```python
from build123d import *

# Parameters (mm, degrees)
F0_R     = 1.85
F0_R_2   = 0.5
F0_W     = 53
F0_H     = 53
F1_DEPTH = 1


with BuildPart() as f1:
    # F0 (on Top) → F1 (new body)
    with BuildSketch(Plane.XY):
        with BuildLine():
            Line((-44, -51), (44, -51))
            ThreePointArc((44, -51), (48.949747, -48.949747), (51, -44))
            Line((51, -44), (51, 44))
            ThreePointArc((51, 44), (48.949747, 48.949747), (44, 51))
            Line((44, 51), (-44, 51))
            ThreePointArc((-44, 51), (-48.949747, 48.949747), (-51, 44))
            Line((-51, 44), (-51, -44))
            ThreePointArc((-51, -44), (-48.949747, -48.949747), (-44, -51))
        make_face()
        with Locations((-41.5, -41.5)):
            Circle(F0_R, mode=Mode.SUBTRACT)
        with Locations((-35.074029, -20.25)):
            Circle(F0_R_2, mode=Mode.SUBTRACT)
        with Locations((41.5, -41.5)):
            Circle(F0_R, mode=Mode.SUBTRACT)
        with Locations((35.074029, -20.25)):
            Circle(F0_R_2, mode=Mode.SUBTRACT)
        with Locations((-41.5, 41.5)):
            Circle(F0_R, mode=Mode.SUBTRACT)
        Rectangle(F0_W, F0_H, mode=Mode.SUBTRACT)
        with Locations((0, 40.5)):
            Circle(F0_R_2, mode=Mode.SUBTRACT)
        with Locations((41.5, 41.5)):
            Circle(F0_R, mode=Mode.SUBTRACT)
    extrude(amount=F1_DEPTH)


solid = f1.part
```
Can you work these out from the model? Positions are in its coordinate system, mm. Coordinates: 2 decimals unless noted, no trailing zeros. Loops run counter-clockwise (first coordinate to the right, second up) from the corner with the lowest first, then second, coordinate; pieces in that order, holes last.
Item 1: If we mould it in two halves opening along Y, with no side actions, what happens to faces 1 (the face through (49, 48.9, 0.5)), 2 (the face through (40.032, 40.374, 0.493)), 3 (the face through (33, 1, 1))? For each: released by +Y, released by -Y, zero draft, split by the parting line, or undercut.
Answers below:
face 1: released by +Y
face 2: undercut
face 3: zero draft
Item 2: Suppose I cut it at C-C (z = 0.75). State how many separate pieces and enclosed holes the cut face has, then the cut area to 3 significant figures.
Answers below:
separate pieces: 1
enclosed holes: 8
area: 7,510 mm2
Item 3: Suppose I cut it at A-A (x = -10.5). Please give me the cut outline in (y, z), then the cut area to 3 significant figures.
Answers below:
outline: (-51, 0) - (-26.5, 0) - (-26.5, 1) - (-51, 1) - close; (26.5, 0) - (51, 0) - (51, 1) - (26.5, 1) - close
area: 49.0 mm2
Item 4: I'm going to push flat-ended pins straight in: pin 1 (2 mm diameter, centred on x = 41.5, y = 41.5, fed in from +Z); pin 2 (6 mm diameter, centred on x = -41.5, y = 41.5, fed in from +Z). Where does each tip first touch, or does it pass through?
Answers below:
pin 1: passes through
pin 2: stops at z = 1
Item 5: Please list where these lines run through material, in increasing order: L1, parallel to Y at x = 41.5, z = 0.5; L2, parallel to X at y = 40.5, z = 0.7; L3, parallel to Y at x = 0, z = 0.8.
Answers below:
L1: y = -51 to -43.35, -39.65 to 39.65, 43.35 to 51
L2: x = -51 to -43.06, -39.94 to -0.5, 0.5 to 39.94, 43.06 to 51
L3: y = -51 to -26.5, 26.5 to 40, 41 to 51
Item 6: Suppose I cut it at D-D (x = 41.5). Please give me the cut outline in (y, z).
Answers below:
outline: (-51, 0) - (-43.35, 0) - (-43.35, 1) - (-51, 1) - close; (-39.65, 0) - (39.65, 0) - (39.65, 1) - (-39.65, 1) - close; (43.35, 0) - (51, 0) - (51, 1) - (43.35, 1) - close
